For this review, take the finished solid that the model builds, in its own axes (mm). Face numbers are marked on the shaded views. A direction names the side the tool comes from. Round coordinates to 2 decimals unless told otherwise and drop trailing zeros. Write each loop counter-clockwise with the first axis right and the second up, starting at its lowest first coordinate (ties: lowest second). Pieces come first, ordered by that corner, then holes. Notation, with made-up numbers: M -33.5,74 L -17.5,74 A16 ccw -17.5,97 Z; hole C -30,15 d4. An arc over 180 degrees is marked long. Answer in a Markdown table with one row per item.
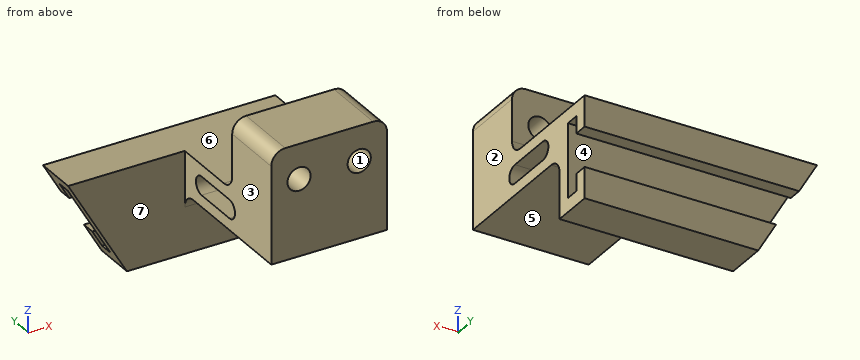
```python
from build123d import *

# Parameters (mm, degrees)
BOSS_EXTRUDE1_DEPTH = 110
CUT_EXTRUDE1_DEPTH  = 155.841854807
SKETCH3_W           = 74.760259453
SKETCH3_H           = 62
CUT_EXTRUDE2_DEPTH  = 155.841854807
SKETCH4_R           = 5
CUT_EXTRUDE3_DEPTH  = 136.132694452
FILLET1_R           = 6


with BuildPart() as part:
    # Sketch1 → Boss-Extrude1 (new body)
    with BuildSketch(Plane(origin=(0, 0, 0), x_dir=(0, 0, -1), z_dir=(1, 0, 0))):
        with BuildLine():
            Line((0, 0), (48, 0))
            Line((48, 0), (48, 56))
            ThreePointArc((48, 56), (49.757359313, 60.242640687), (54, 62))
            Line((54, 62), (74, 62))
            Line((74, 62), (74, 80))
            Line((74, 80), (60.615384615, 80))
            Line((60.615384615, 80), (60.615384615, 74))
            Line((60.615384615, 74), (68, 74))
            Line((68, 74), (68, 68))
            Line((68, 68), (36, 68))
            Line((36, 68), (36, 74))
            Line((36, 74), (43.384615385, 74))
            Line((43.384615385, 74), (43.384615385, 80))
            Line((43.384615385, 80), (30, 80))
            Line((30, 80), (30, 34))
            ThreePointArc((30, 34), (28.242640687, 29.757359313), (24, 28))
            Line((24, 28), (0, 28))
            Line((0, 28), (0, 0))
        make_face()
        with BuildLine():
            Line((43, 50), (43, 30))
            ThreePointArc((43, 30), (39, 26), (35, 30))
            Line((35, 30), (35, 50))
            ThreePointArc((35, 50), (39, 54), (43, 50))
        make_face(mode=Mode.SUBTRACT)
    extrude(amount=-BOSS_EXTRUDE1_DEPTH)

    # Sketch2 → Cut-Extrude1 (cut, through all)
    with BuildSketch(Plane(origin=(0, 80, 0), x_dir=(1, 0, 0), z_dir=(0, 1, 0))):
        Polygon((-110, 74), (-110, 13.378221735), (-75, 74), align=None)
    extrude(amount=-CUT_EXTRUDE1_DEPTH, mode=Mode.SUBTRACT)

    # Sketch3 → Cut-Extrude2 (cut, through all)
    with BuildSketch(Plane.XY):
        with Locations((-87.380129727, 31)):
            Rectangle(SKETCH3_W, SKETCH3_H)
    extrude(amount=-CUT_EXTRUDE2_DEPTH, mode=Mode.SUBTRACT)

    # Sketch4 → Cut-Extrude3 (cut, through all)
    with BuildSketch(Plane(origin=(0, 28, 0), x_dir=(1, 0, 0), z_dir=(0, 1, 0))):
        with Locations(Location((-38, 15, 0), (0, 0, 270))):
            Circle(SKETCH4_R)
        with Locations(Location((-12, 15, 0), (0, 0, 270))):
            Circle(SKETCH4_R)
    extrude(amount=-CUT_EXTRUDE3_DEPTH, mode=Mode.SUBTRACT)

    # Fillet1
    fillet1_edges = [part.edges().sort_by_distance(p)[0] for p in [
        (-50, 14, 0),
        (0, 14, 0),
    ]]
    fillet(fillet1_edges, radius=FILLET1_R)


solid = part.part
```
Q1. Insertion check: P1, Ø1, axis at x = -19, y = 69, coming from the +Z side; P2, Ø15, axis at x = -35, y = 30.5, coming from the -Z side; P3, Ø1.5, axis at x = -61, z = -57.5, coming from the -Y side. Each pin has a flat end and moves straight along its axis. Give the tip position at first contact, or say it passes through.
Found:
| item | result |
|---|---|
| P1 | z = -30 |
| P2 | z = -48 |
| P3 | y = 62 |
Q2. Take a section at D-D (z = -65.5). State the section outline as (x, y) points, then the cut area to 3 significant figures.
Found:
| item | result |
|---|---|
| outline | M -79.91,62 L 0,62 L 0,68 L -79.91,68 Z; M -79.91,74 L 0,74 L 0,80 L -79.91,80 Z |
| area | 959 mm² |
Q3. For probe 1 along X at (y, z) = (9, -15); probe 2 along Y at (x, z) = (-22.5, -10.5); probe 3 along Y at (x, z) = (-79.5, -43), list the stretches that pass through material, from the lowest coordinate up.
Found:
| item | result |
|---|---|
| probe 1 | -50 to -43, -33 to -17, -7 to 0 |
| probe 2 | 0 to 28 |
| probe 3 | 62 to 68, 74 to 80 |
Q4. Take a section at C-C (y = 12.5). State the section outline as (x, z) points.
Found:
| item | result |
|---|---|
| outline | M -50,-48 L 0,-48 L 0,-6 A6 ccw -6,0 L -44,0 A6 ccw -50,-6 Z; hole C -38,-15 d10; hole C -12,-15 d10 |
Q5. Machinability: for the marked faces 4, 5, 6 and 7, which of the approach directions +Z, -Z, +X, -X, +Y, -Y give a long, thin tool a straight path to every point of the face, cutting with its end or side? Answer none if there is none.
Found:
| item | result |
|---|---|
| face 4 | +X, -X |
| face 5 | -Z, +X, -X, -Y |
| face 6 | +Z, +X, -X, +Y |
| face 7 | -Z, -X, -Y |
Q6. Take a section at A-A (x = -12). State the section outline as (y, z) points, then the cut area to 3 significant figures.
Found:
| item | result |
|---|---|
| outline | M 0,-48 L 56,-48 A6 cw 62,-54 L 62,-74 L 80,-74 L 80,-60.62 L 74,-60.62 L 74,-68 L 68,-68 L 68,-36 L 74,-36 L 74,-43.38 L 80,-43.38 L 80,-30 L 34,-30 A6 cw 28,-24 L 28,-20 L 0,-20 Z; M 0,-10 L 28,-10 L 28,0 L 0,0 Z; hole M 30,-43 L 50,-43 A4 ccw 50,-35 L 30,-35 A4 ccw Z |
| area | 1,980 mm² |
Q7. Mouldability with a two-part tool opening along X and no side actions: class the marked faces 1, 2 and 3 as +X half, -X half, draft (parallel to the pull), parting line (faces both ways), or undercut.
Found:
| item | result |
|---|---|
| face 1 | undercut |
| face 2 | +X half |
| face 3 | -X half |
Q8. Take a section at B-B (z = -15). State the section outline as (x, y) points, then the cut area to 3 significant figures.
Found:
| item | result |
|---|---|
| outline | M -50,0 L -43,0 L -43,28 L -50,28 Z; M -33,0 L -17,0 L -17,28 L -33,28 Z; M -7,0 L 0,0 L 0,28 L -7,28 Z |
| area | 840 mm² |
